Geometry check sheet. Reference: the model listing, model coordinates, mm. A direction names the side the tool comes from. Coordinates: 2 decimals unless noted, no trailing zeros. Loops run counter-clockwise (first coordinate to the right, second up) from the corner with the lowest first, then second, coordinate; pieces in that order, holes last. Notation, with made-up numbers: M -7.5,54 L 26.5,54 A29 cw 26.5,79 Z; hole C 60.5,33.5 d1. An arc over 180 degrees is marked long. Use CSV: the item, a comma, the result in double quotes.
```python
from build123d import *

# Parameters (mm, degrees)
BOSS_EXTRUDE3_DEPTH = 1.1
BOSS_EXTRUDE4_DEPTH = 24
BOSS_EXTRUDE5_DEPTH = 5.7
BOSS_EXTRUDE6_DEPTH = 6.95
SKETCH8_R           = 2.41
BOSS_EXTRUDE7_DEPTH = 9.7
BOSS_EXTRUDE8_DEPTH = 2


# Read off the part's stored shape, not the designer's step: Imported1
with BuildPart() as part:
    # Sketch4 → Boss-Extrude3 (new body)
    with BuildSketch(Plane(origin=(0, 11.6, 0), x_dir=(1, 0, 0), z_dir=(0, 1, 0))):
        with BuildLine():
            Line((-32.298673735, 38.799155683), (-7.398673735, 38.799155683))
            ThreePointArc((-7.398673735, 38.799155683), (-6.448673735, 37.849155683), (-7.398673735, 36.899155683))
            Line((-7.398673735, 36.899155683), (-8.348673735, 36.899155683))
            Line((-8.348673735, 36.899155683), (-8.348673735, 28.699155683))
            Line((-8.348673735, 28.699155683), (-7.398673735, 28.699155683))
            ThreePointArc((-7.398673735, 28.699155683), (-6.448673735, 27.749155683), (-7.398673735, 26.799155683))
            Line((-7.398673735, 26.799155683), (-32.298673735, 26.799155683))
            ThreePointArc((-32.298673735, 26.799155683), (-33.248673735, 27.749155683), (-32.298673735, 28.699155683))
            Line((-32.298673735, 28.699155683), (-31.348673735, 28.699155683))
            Line((-31.348673735, 28.699155683), (-31.348673735, 36.899155683))
            Line((-31.348673735, 36.899155683), (-32.298673735, 36.899155683))
            ThreePointArc((-32.298673735, 36.899155683), (-33.248673735, 37.849155683), (-32.298673735, 38.799155683))
        make_face()
    extrude(amount=BOSS_EXTRUDE3_DEPTH)

    # Sketch5 → Boss-Extrude4 (add)
    with BuildSketch(Plane(origin=(0, 10.5, 0), x_dir=(1, 0, 0), z_dir=(0, 1, 0))):
        with BuildLine():
            Line((-31.348673735, 27.299155683), (-31.348673735, 38.299155683))
            ThreePointArc((-31.348673735, 38.299155683), (-31.202227125, 38.652709074), (-30.848673735, 38.799155683))
            Line((-30.848673735, 38.799155683), (-8.848673735, 38.799155683))
            ThreePointArc((-8.848673735, 38.799155683), (-8.495120344, 38.652709074), (-8.348673735, 38.299155683))
            Line((-8.348673735, 38.299155683), (-8.348673735, 27.299155683))
            ThreePointArc((-8.348673735, 27.299155683), (-8.495120344, 26.945602293), (-8.848673735, 26.799155683))
            Line((-8.848673735, 26.799155683), (-30.848673735, 26.799155683))
            ThreePointArc((-30.848673735, 26.799155683), (-31.202227125, 26.945602293), (-31.348673735, 27.299155683))
        make_face()
    extrude(amount=BOSS_EXTRUDE4_DEPTH)

    # Sketch6 → Boss-Extrude5 (add)
    with BuildSketch(Plane(origin=(0, 7, 0), x_dir=(1, 0, 0), z_dir=(0, 1, 0))):
        with BuildLine():
            Line((-19.448673735, 29.799155683), (-20.268319416, 29.799155683))
            ThreePointArc((-20.268319416, 29.799155683), (-31.248673735, 32.799155683), (-20.268319416, 35.799155683))
            Line((-20.268319416, 35.799155683), (-19.448673735, 35.799155683))
            ThreePointArc((-19.448673735, 35.799155683), (-16.448673735, 32.799155683), (-19.448673735, 29.799155683))
        make_face()
    extrude(amount=BOSS_EXTRUDE5_DEPTH)

    # Sketch7 → Boss-Extrude6 (add)
    with BuildSketch(Plane(origin=(0, 5.75, 0), x_dir=(1, 0, 0), z_dir=(0, 1, 0))):
        with BuildLine():
            Line((-19.448673735, 34.049155683), (-20.869834599, 34.049155683))
            ThreePointArc((-20.869834599, 34.049155683), (-29.998673735, 32.799155683), (-20.869834599, 31.549155683))
            Line((-20.869834599, 31.549155683), (-19.448673735, 31.549155683))
            ThreePointArc((-19.448673735, 31.549155683), (-18.198673735, 32.799155683), (-19.448673735, 34.049155683))
        make_face()
    extrude(amount=BOSS_EXTRUDE6_DEPTH)

    # Sketch8 → Boss-Extrude7 (add)
    with BuildSketch(Plane(origin=(0, 3, 0), x_dir=(1, 0, 0), z_dir=(0, 1, 0))):
        with Locations(Location((-25.348673735, 32.799155683, 0), (0, 0, 270))):
            Circle(SKETCH8_R)
    extrude(amount=BOSS_EXTRUDE7_DEPTH)

    # Sketch1 → Boss-Extrude8 (add)
    with BuildSketch(Plane(origin=(0, 12.7, 0), x_dir=(1, 0, 0), z_dir=(0, 1, 0))):
        with BuildLine():
            Line((-34.948673735, 38.799155683), (-4.748673735, 38.799155683))
            ThreePointArc((-4.748673735, 38.799155683), (-4.112277632, 38.535551786), (-3.848673735, 37.899155683))
            Line((-3.848673735, 37.899155683), (-3.848673735, 34.401497719))
            ThreePointArc((-3.848673735, 34.401497719), (-4.035902323, 34.123500221), (-4.363891126, 34.192496584))
            ThreePointArc((-4.363891126, 34.192496584), (-7.798673735, 32.799155683), (-4.363891126, 31.405814782))
            ThreePointArc((-4.363891126, 31.405814782), (-4.035902323, 31.474811145), (-3.848673735, 31.196813647))
            Line((-3.848673735, 31.196813647), (-3.848673735, 27.699155683))
            ThreePointArc((-3.848673735, 27.699155683), (-4.112277632, 27.06275958), (-4.748673735, 26.799155683))
            Line((-4.748673735, 26.799155683), (-34.948673735, 26.799155683))
            ThreePointArc((-34.948673735, 26.799155683), (-35.585069838, 27.06275958), (-35.848673735, 27.699155683))
            Line((-35.848673735, 27.699155683), (-35.848673735, 31.196813647))
            ThreePointArc((-35.848673735, 31.196813647), (-35.661445146, 31.474811145), (-35.333456343, 31.405814782))
            ThreePointArc((-35.333456343, 31.405814782), (-31.898673735, 32.799155683), (-35.333456343, 34.192496584))
            ThreePointArc((-35.333456343, 34.192496584), (-35.661445146, 34.123500221), (-35.848673735, 34.401497719))
            Line((-35.848673735, 34.401497719), (-35.848673735, 37.899155683))
            ThreePointArc((-35.848673735, 37.899155683), (-35.585069838, 38.535551786), (-34.948673735, 38.799155683))
        make_face()
    extrude(amount=BOSS_EXTRUDE8_DEPTH)


solid = part.part
```
1. Section check D-D, the plane x = -17. Record the cut outline in (y, z).
The answers:
outline,"M 7,-34.53 L 10.5,-34.53 L 10.5,-38.8 L 34.5,-38.8 L 34.5,-26.8 L 10.5,-26.8 L 10.5,-31.07 L 7,-31.07 Z"
2. Section check C-C, the plane x = -29. Record the cut outline in (y, z), plus the area to 3 significant figures.
The answers:
outline,"M 5.75,-35.68 L 7,-35.68 L 7,-37.43 L 10.5,-37.43 L 10.5,-38.8 L 34.5,-38.8 L 34.5,-26.8 L 10.5,-26.8 L 10.5,-28.16 L 7,-28.16 L 7,-29.92 L 5.75,-29.92 Z"
area,"328 mm^2"
3. Set-up check for faces 1 (the flat face through (-32, 12, -36.899)), 2 (the flat face through (-24, 5.75, -35)), 3 (the flat face through (-31.349, 24, -33)), 4 (the flat face through (-8.349, 24, -33)): record each of +Z, -Z, +X, -X, +Y, -Y from which the full face is reachable in a straight line by a thin tool's end or side.
The answers:
face 1,"-X, -Y"
face 2,"-Y"
face 3,"+Z, -Z, -X, +Y"
face 4,"+Z, -Z, +X, +Y"
4. Release check for a two-part mould opening along Z. For faces 5 (the flat face through (-31.349, 12, -33)), 6 (the cylindrical face through (-16.45, 8.73, -32.87)), 7 (the flat face through (-20, 22, -38.799)) record: +Z half, -Z half, draft (parallel to the pull), parting line (faces both ways), or undercut.
The answers:
face 5,"undercut"
face 6,"parting line"
face 7,"-Z half"
5. Section check A-A, the plane y = 27.5. Record the cut outline in (x, z), plus the area to 3 significant figures.
The answers:
outline,"M -31.35,-38.3 A0.5 ccw -30.85,-38.8 L -8.85,-38.8 A0.5 ccw -8.35,-38.3 L -8.35,-27.3 A0.5 ccw -8.85,-26.8 L -30.85,-26.8 A0.5 ccw -31.35,-27.3 Z"
area,"276 mm^2"
6. Thickness scan on line 1 (X direction, y = 22.5, z = -32.5); line 2 (Y direction, x = -25.5, z = -37); line 3 (Y direction, x = -7.5, z = -35). Record the ranges inside material, lowest first. Write a range as [from, to].
The answers:
line 1,"[-31.35, -8.35]"
line 2,"[5.75, 34.5]"
line 3,"[12.7, 14.7]"
7. Section check B-B, the plane z = -32.25. Record the cut outline in (x, y).
The answers:
outline,"M -31.98,12.7 L -31.35,12.7 L -31.35,10.5 L -31.22,10.5 L -31.22,7 L -29.97,7 L -29.97,5.75 L -27.7,5.75 L -27.7,3 L -23,3 L -23,5.75 L -18.33,5.75 L -18.33,7 L -16.5,7 L -16.5,10.5 L -8.35,10.5 L -8.35,12.7 L -7.72,12.7 L -7.72,14.7 L -8.35,14.7 L -8.35,34.5 L -31.35,34.5 L -31.35,14.7 L -31.98,14.7 Z"
8. Gauge pin test, flat ends, axial feed: P1, Ø5, axis at x = -32.5, z = -35.5, coming from the -Y side; P2, Ø1.1, axis at y = 11.5, z = -30.5, coming from the +X side; P3, Ø0.7, axis at x = -19.5, y = 9, coming from the -Z side. Record the tip position at first contact, or that the pin passes through.
The answers:
P1,"y = 7"
P2,"x = -8.35"
P3,"z = -35.8"
